Autodesk Inventor part; units mm, degrees
ref_plane "YZ Plane" through (0, 0, 0) normal (1, 0, 0) x (0, 1, 0)
ref_plane "XZ Plane" through (0, 0, 0) normal (0, 1, 0) x (-1, 0, 0)
ref_plane "XY Plane" through (0, 0, 0) normal (0, 0, 1) x (1, 0, 0)
sketch "Sketch1" plane through (0, 0, 0) normal (0, 1, 0) x (-1, 0, 0)
  line L0 (-4.9075, -8.5) -> (-9.815, 0)
  line L1 (-9.815, 0) -> (-4.9075, 8.5)
  line L2 (-4.9075, 8.5) -> (4.9075, 8.5)
  line L3 (4.9075, 8.5) -> (9.815, 0)
  line L4 (9.815, 0) -> (4.9075, -8.5)
  line L5 (4.9075, -8.5) -> (-4.9075, -8.5)
  point P0 (0, 0)
  point P1 (0, 0)
  dimension "d0" = 17
extrude "Extrusion1" add sketch "Sketch1" along normal blind 20
ref_plane "Work Plane1" through (0, 60, 0) normal (0, 1, 0) x (1, 0, 0)
sketch "Sketch2" plane through (0, 60, 0) normal (0, 1, 0) x (1, 0, 0)
  point P0 (0, 0)
  point P1 (0, 0)
loft "Loft1" add section 1 edges at (-7.3612, 20, -4.25) (-7.3612, 20, 4.25) (0, 20, 8.5) (7.3612, 20, 4.25) (7.3612, 20, -4.25) (0, 20, -8.5) section 2 point at (0, 60, 0)
properties part number "Punta caibración_3DPrint"
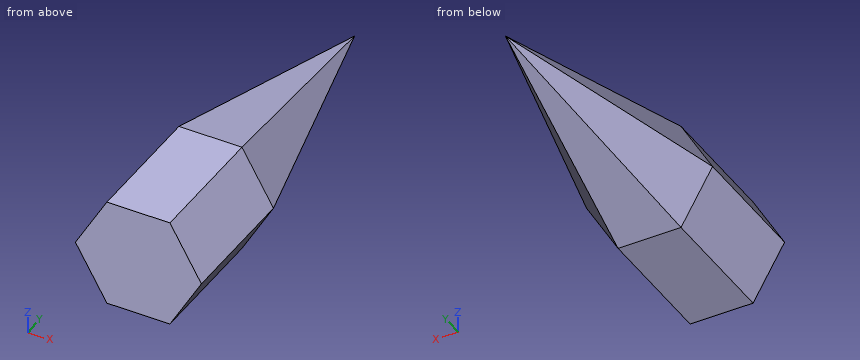
Geometry: final body of the model. Coordinates: model frame, mm. Give positions to 0.01 mm unless a question says otherwise; leave off trailing zeros. Write each loop counter-clockwise with the first axis right and the second up, starting at its lowest first coordinate (ties: lowest second). Pieces come first, ordered by that corner, then holes. Notation, with made-up numbers: M 22,52 L 53,52 A19 cw 53,75 Z; hole C -33,89.25 d6. An arc over 180 degrees is marked long. Answer in a Markdown table with one row per item. Add a question column.
(1) Section B-B on x = 4. Return loops of the section in (y, z).
(2) Section C-C on z = 3.75. Return loops of the section in (x, y), and give its area (3 significant figures).
(3) Section A-A on y = 7. Return loops of the section in (x, z) (1 decimal), and give its area (3 significant figures).
(4) Ray query, line 1 (X direction, y = 43, z = -0.75); line 2 (X direction, y = 32, z = 3.5); line 3 (Z direction, x = 3, y = 34.5). Return the intervals inside material, ascending.
(5) Section D-D on x = 0.75. Return loops of the section in (y, z).
(6) First-contact query: pin 1 (10 mm diameter, centred on x = -2, y = 27.5, fed in from -Z); pin 2 (4 mm diameter, centred on x = 2, y = 47.5, fed in from +Z); pin 3 (4 mm diameter, centred on y = 46, z = -3.5, fed in from -X). Flat tips, straight axial feed; report the tip coordinate or a pass-through.
Result set:
| question | item | result |
|---|---|---|
| 1 | outline | M 0,-8.5 L 20,-8.5 L 27.4,-6.93 L 43.7,0 L 27.4,6.93 L 20,8.5 L 0,8.5 Z |
| 2 | outline | M -7.65,0 L 7.65,0 L 7.65,20 L 2.17,42.35 L -2.17,42.35 L -7.65,20 Z |
| 2 | area | 525 mm^2 |
| 3 | outline | M -9.8,0 L -4.9,-8.5 L 4.9,-8.5 L 9.8,0 L 4.9,8.5 L -4.9,8.5 Z |
| 3 | area | 250 mm^2 |
| 4 | line 1 | x = -3.74 to 3.74 |
| 4 | line 2 | x = -4.85 to 4.85 |
| 4 | line 3 | z = -5.42 to 5.42 |
| 5 | outline | M 0,-8.5 L 20,-8.5 L 53.89,-1.3 L 56.94,0 L 53.89,1.3 L 20,8.5 L 0,8.5 Z |
| 6 | pin 1 | stops at z = -7.97 |
| 6 | pin 2 | stops at z = 3.08 |
| 6 | pin 3 | stops at x = -2.67 |
